Check sheet for the modelled part. Datum: model origin and axes. Units: mm. A direction names the side the tool comes from. Coordinates: 2 decimals unless noted, no trailing zeros. Loops run counter-clockwise (first coordinate to the right, second up) from the corner with the lowest first, then second, coordinate; pieces in that order, holes last. Notation, with made-up numbers: (-28.75, 59) - (-1.75, 59) arc R16 ccw to (-1.75, 70) - close; hole circle Ø4 at (45, 65). An arc over 180 degrees is marked (long way). Use a Markdown table: item, result. Add a question column.
1) Thickness scan on line 1 (Z direction, x = 7.25, y = 2.75); line 2 (Y direction, x = 1.75, z = 3); line 3 (Z direction, x = 5, y = -5.5). Record the ranges inside material, lowest first.
2) Sectioned sample at C-C, the plane y = -6.5. Enter the section's corners in (x, z).
3) Sectioned sample at A-A, the plane y = 0. Enter the section's corners in (x, z), then the cut area to 3 significant figures.
4) Sectioned sample at B-B, the plane x = 8.5. Enter the section's corners in (y, z).
5) Tool access check on faces 1 (the flat face through (10, -2, -5)), 2 (the cylindrical face through (7.1, -6.75, -0.09)). Record the directions out of +Z, -Z, +X, -X, +Y, -Y that give a thin tool (end or side, any length) a straight path to the whole face; none if there is none.
6) Draft check along Z on faces 3 (the flat face through (0, -2, -5)), 4 (the cylindrical face through (5.056, 3.966, 0.521)), 5 (the cylindrical face through (5.07, 3, -9.54)). Enter one of: pulls with the +Z half, pulls with the -Z half, needs draft (parallel to the pull), parting line crosses it, or undercut.
7) Sectioned sample at D-D, the plane z = 1. State how many separate pieces and enclosed holes the cut face has, then the cut area to 3 significant figures.
from build123d import *

# Parameters (mm, degrees)
SKETCH1_W                 = 10
SKETCH1_H                 = 10
F_8_0_8_DIAMETER_HOLE1_D  = 8
M5X0_8_TAPPED_HOLE1_D     = 4.2
M5X0_8_TAPPED_HOLE1_DEPTH = 6.59617233
CHAMFER1_SIZE             = 1


with BuildPart() as part:
    # Sketch1 → Revolve1 (revolve)
    with BuildSketch(Plane.XY, mode=Mode.PRIVATE) as revolve1_sk:
        with Locations((5, 5)):
            Rectangle(SKETCH1_W, SKETCH1_H)
    revolve(revolve1_sk.sketch.rotate(Axis((0, 0, 0), (1, 0, 0)), 270), axis=Axis((0, 0, 0), (1, 0, 0)))

    # Ø8.0 (8) Diameter Hole1 (through all)
    with Locations(Plane.ZY):
        with Locations((0, 0)):
            Hole(F_8_0_8_DIAMETER_HOLE1_D / 2)

    # M5x0.8 Tapped Hole1
    with Locations(Plane(origin=(0, -3.40382767, 0), x_dir=(1, 0, 0), z_dir=(0, 1, 0))):
        with Locations((5, 0.000941977)):
            Hole(M5X0_8_TAPPED_HOLE1_D / 2, depth=M5X0_8_TAPPED_HOLE1_DEPTH)

    # Chamfer1
    chamfer1_edges = [part.edges().sort_by_distance(p)[0] for p in [
        (0, 0, 4),
        (10, 0, 4),
    ]]
    chamfer(chamfer1_edges, length=CHAMFER1_SIZE)


solid = part.part
Solved:
| question | item | result |
|---|---|---|
| 1 | line 1 | z = -9.61 to -2.9, 2.9 to 9.61 |
| 1 | line 2 | y = -9.54 to -2.65, 2.65 to 9.54 |
| 1 | line 3 | z = -8.35 to -2.1, 2.1 to 8.35 |
| 2 | outline | (0, -7.6) - (10, -7.6) - (10, 7.6) - (0, 7.6) - close; hole circle Ø4.2 at (5, 0) |
| 3 | outline | (0, -10) - (10, -10) - (10, -5) - (9, -4) - (1, -4) - (0, -5) - close; (0, 5) - (1, 4) - (9, 4) - (10, 5) - (10, 10) - (0, 10) - close |
| 3 | area | 118 mm2 |
| 4 | outline | circle Ø20 at (0, 0); hole circle Ø8 at (0, 0) |
| 5 | face 1 | +Z, -Z, +X, +Y, -Y |
| 5 | face 2 | -Y |
| 6 | face 3 | needs draft |
| 6 | face 4 | undercut |
| 6 | face 5 | parting line crosses it |
| 7 | separate pieces | 3 |
| 7 | enclosed holes | 0 |
| 7 | area | 97.0 mm2 |
